Autodesk Inventor part; units mm, degrees
ref_plane "우측면도" through (0, 0, 0) normal (1, 0, 0) x (0, 1, 0)
ref_plane "평면도" through (0, 0, 0) normal (0, 1, 0) x (-1, 0, 0)
ref_plane "정면도" through (0, 0, 0) normal (0, 0, 1) x (1, 0, 0)
sketch "스케치1" plane through (0, 0, 0) normal (0, 1, 0) x (-1, 0, 0)
  line L0 (-16, 71) -> (16, 71)
  line L1 (16, 71) -> (16, -71)
  line L2 (16, -71) -> (-16, -71)
  line L3 (-16, -71) -> (-16, 71)
  line L4 (-16, 71) -> (16, -71) construction
  line L5 (16, 71) -> (-16, -71) construction
  line L6 (-16, -71) -> (-4, -71)
  line L7 (-4, -71) -> (-4, -77)
  line L8 (-4, -77) -> (-16, -77)
  line L9 (-16, -77) -> (-16, -71)
  line L10 (-16, 71) -> (-4, 71)
  line L11 (-4, 71) -> (-4, 77)
  line L12 (-4, 77) -> (-16, 77)
  line L13 (-16, 77) -> (-16, 71)
  point P0 (0, 0)
  dimension "d0" = 32
  dimension "d1" = 142
  dimension "d2" = 12
  dimension "d3" = 6
  dimension "d4" = 12
  dimension "d5" = 6
extrude "돌출1" add sketch "스케치1" along normal blind 6
sketch "스케치2" plane through (0, 6, 0) normal (0, 1, 0) x (1, 0, 0)
  line L0 (-5, -40) -> (5, -40)
  line L1 (5, -40) -> (5, 40)
  line L2 (5, 40) -> (-5, 40)
  line L3 (-5, 40) -> (-5, -40)
  line L4 (-5, -40) -> (5, 40) construction
  line L5 (5, -40) -> (-5, 40) construction
  point P0 (0, 0)
  dimension "d8" = 10
  dimension "d9" = 80
extrude "돌출2" cut sketch "스케치2" against normal blind 6
sketch "스케치3" plane through (0, 6, 0) normal (0, 1, 0) x (1, 0, 0)
  line L0 (-5, 40) -> (5, 40)
  line L1 (5, 40) -> (5, -40)
  line L2 (5, -40) -> (-5, -40)
  line L3 (-5, -40) -> (-5, 40)
  line L4 (-16, -71) -> (4, -71)
  line L5 (4, -71) -> (4, -77)
  line L6 (4, -77) -> (16, -77)
  line L7 (16, -77) -> (16, 77)
  line L8 (16, 77) -> (4, 77)
  line L9 (4, 77) -> (4, 71)
  line L10 (4, 71) -> (-16, 71)
  line L11 (-16, 71) -> (-16, -71)
  circle A0 centre (4, -71) radius 1
  circle A1 centre (4, 71) radius 1
  point P0 (0, 0)
  dimension "d12" = 2
  dimension "d13" = 2
extrude "돌출3" cut sketch "스케치3" against normal through all contours A0 L5 L4 | L4 L5 A0 | A1 L9 L10 | L10 L9 A1
properties part number "battery bottomplate" material "PMMA 플라스틱"
The model under review builds one solid part; all positions refer to its coordinate system, in mm. A direction names the side the tool comes from. Round coordinates to 2 decimals unless told otherwise and drop trailing zeros. Order: outer loops, then holes, each group sorted by start corner. A loop starts at its lowest first (then second) coordinate and runs counter-clockwise, first axis right, second up. Notation, with made-up numbers: (20, 1) -> (67, 1) arc R18 ccw to (67, 28) -> close; hole circle Ø10 at (34.25, 3). An arc over 180 degrees is marked (long way). Use CSV: the item, a comma, the result in double quotes. Start each with the question number.
(1) Mouldability with a two-part tool opening along X and no side actions: class faces 4 (the face through (-7, 3, -71)), 5 (the face through (5, 3, 1)), 6 (the face through (16, 3, 1)) as pulls with the +X half, pulls with the -X half, needs draft (parallel to the pull), parting line crosses it, or undercut.
(2) Wall thickness on probe 1 along X at (y, z) = (3.5, -32.5); probe 2 along Z at (x, y) = (0, 2.65); probe 3 along Z at (x, y) = (-7, 0.5): over which ranges is each line inside the solid? List them lowest first. Write a range as from..to.
(3) Tool access review of faces 1 (the face through (4, 3, 74)), 2 (the face through (4, 3, -74)), 3 (the face through (-5, 3, -1)): name each direction out of +Z, -Z, +X, -X, +Y, -Y from which nothing blocks a thin tool from reaching the whole face with its end or side.
(4) Insertion check: pin 1 (3 mm diameter, centred on x = -3.5, y = 4, fed in from -Z); pin 2 (1.8 mm diameter, centred on x = 0.5, y = 4, fed in from +Z). Each pin has a flat end and moves straight along its axis. Give the tip position at first contact, or say it passes through.
(5) Consider section A-A on z = 23. Write out the cut boundary in (x, y).
(6) Consider section B-B on y = 3.65. Write out the cut boundary in (x, z), and give its area (3 significant figures).
Responses:
1,face 4,"needs draft"
1,face 5,"undercut"
1,face 6,"pulls with the +X half"
2,probe 1,"-16..-5, 5..16"
2,probe 2,"-71..-40, 40..71"
2,probe 3,"-71..71"
3,face 1,"+Z, -X, +Y, -Y"
3,face 2,"-Z, -X, +Y, -Y"
3,face 3,"+Y, -Y"
4,pin 1,"z = -71"
4,pin 2,"z = 71"
5,outline,"(-16, 0) -> (-5, 0) -> (-5, 6) -> (-16, 6) -> close; (5, 0) -> (16, 0) -> (16, 6) -> (5, 6) -> close"
6,outline,"(-16, -71) -> (3, -71) arc R1 cw (long way) to (4, -72) -> (4, -77) -> (16, -77) -> (16, 77) -> (4, 77) -> (4, 72) arc R1 cw (long way) to (3, 71) -> (-16, 71) -> close; hole (-5, -40) -> (5, -40) -> (5, 40) -> (-5, 40) -> close"
6,area,"3,880 mm²"
